```python
from build123d import *

# Parameters (mm, degrees)
F1_DEPTH      = 400
F2_W          = 150
F2_H          = 5
F2_W_2        = 75
F3_DEPTH      = 645
F4_W          = 2.5
F4_H          = 50
F5_DEPTH      = 21
F6_R          = 2
F8_DEPTH      = 143
F8_DEPTH_BACK = 143
F9_R          = 2


with BuildPart() as f1:
    # F0 (on Front) → F1 (new body)
    with BuildSketch(Plane.XZ):
        with BuildLine():
            ThreePointArc((150, 73), (148.6819805153, 76.1819805153), (145.5, 77.5))
            Line((145.5, 77.5), (0, 77.5))
            Line((0, 77.5), (-145.5, 77.5))
            ThreePointArc((-145.5, 77.5), (-148.6819805153, 76.1819805153), (-150, 73))
            Line((-150, 73), (-150, 25.5))
            ThreePointArc((-150, 25.5), (-149.7286167935, 23.960909355), (-148.947199994, 22.6074557564))
            Line((-148.947199994, 22.6074557564), (-148.5848888922, 22.1756701992))
            ThreePointArc((-148.5848888922, 22.1756701992), (-148.150768448, 21.4237515333), (-148, 20.5687011749))
            Line((-148, 20.5687011749), (-148, -77.5))
            Line((-148, -77.5), (-146, -77.5))
            Line((-146, -77.5), (-146, 20.5687011749))
            ThreePointArc((-146, 20.5687011749), (-146.2713832065, 22.1077918199), (-147.052800006, 23.4612454185))
            Line((-147.052800006, 23.4612454185), (-147.4151111078, 23.8930309758))
            ThreePointArc((-147.4151111078, 23.8930309758), (-147.849231552, 24.6449496417), (-148, 25.5))
            Line((-148, 25.5), (-148, 73))
            ThreePointArc((-148, 73), (-147.267766953, 74.767766953), (-145.5, 75.5))
            Line((-145.5, 75.5), (0, 75.5))
            Line((0, 75.5), (145.5, 75.5))
            ThreePointArc((145.5, 75.5), (147.267766953, 74.767766953), (148, 73))
            Line((148, 73), (148, 25.5))
            ThreePointArc((148, 25.5), (147.849231552, 24.6449496417), (147.4151111078, 23.8930309758))
            Line((147.4151111078, 23.8930309758), (147.052800006, 23.4612454185))
            ThreePointArc((147.052800006, 23.4612454185), (146.2713832065, 22.1077918199), (146, 20.5687011749))
            Line((146, 20.5687011749), (146, -77.5))
            Line((146, -77.5), (148, -77.5))
            Line((148, -77.5), (148, 20.5687011749))
            ThreePointArc((148, 20.5687011749), (148.150768448, 21.4237515333), (148.5848888922, 22.1756701992))
            Line((148.5848888922, 22.1756701992), (148.947199994, 22.6074557564))
            ThreePointArc((148.947199994, 22.6074557564), (149.7286167935, 23.960909355), (150, 25.5))
            Line((150, 25.5), (150, 73))
        make_face()
    extrude(amount=F1_DEPTH)

    # F2 (on face) → F3 (cut)
    with BuildSketch(Plane.YZ.offset(148)):
        with Locations((-200, -75)):
            Rectangle(F2_W, F2_H)
        with Locations((-37.5, -75)):
            Rectangle(F2_W_2, F2_H)
        with Locations((-362.5, -75)):
            Rectangle(F2_W_2, F2_H)
    extrude(amount=-F3_DEPTH, mode=Mode.SUBTRACT)

    # F4 (on face) → F5 (cut)
    with BuildSketch(Plane.XY.offset(77.5)):
        with Locations((146.75, -100)):
            Rectangle(F4_W, F4_H)
        with Locations((146.75, -300)):
            Rectangle(F4_W, F4_H)
        with Locations((-146.75, -100)):
            Rectangle(F4_W, F4_H)
        with Locations((-146.75, -300)):
            Rectangle(F4_W, F4_H)
    extrude(amount=-F5_DEPTH, mode=Mode.SUBTRACT)

    # F6
    f6_edges = [f1.edges().sort_by_distance(p)[0] for p in [
        (147, -125, -72.5),
        (147, -325, -72.5),
        (-147, -325, -72.5),
        (-147, -125, -72.5),
        (147, -75, -72.5),
        (147, -275, -72.5),
        (-147, -275, -72.5),
        (-147, -75, -72.5),
        (147, -325, -77.5),
        (147, -125, -77.5),
        (-147, -325, -77.5),
        (-147, -125, -77.5),
        (147, -275, -77.5),
        (147, -75, -77.5),
        (-147, -275, -77.5),
        (-147, -75, -77.5),
    ]]
    fillet(f6_edges, radius=F6_R)

    # F7 (on Right) → F8 (join, two sides)
    with BuildSketch(Plane.YZ) as f8_sk:
        with BuildLine():
            Line((1, 77.5), (0, 77.5))
            Line((0, 77.5), (0, 75.5))
            Line((0, 75.5), (1, 75.5))
            ThreePointArc((1, 75.5), (2.767766953, 74.767766953), (3.5, 73))
            Line((3.5, 73), (3.5, 72))
            Line((3.5, 72), (5.5, 72))
            Line((5.5, 72), (5.5, 73))
            ThreePointArc((5.5, 73), (4.1819805153, 76.1819805153), (1, 77.5))
        make_face()
    extrude(amount=F8_DEPTH)
    extrude(f8_sk.sketch, amount=-F8_DEPTH_BACK)

    # F9 (call 1 of 4: OpenCascade refuses the feature's edges together)
    f9_edges = [f1.edges().sort_by_distance(p)[0] for p in [
        (143, 0, 76.5),
    ]]
    fillet(f9_edges, radius=F9_R)

    # F9#2 (call 2 of 4)
    f9_2_edges = [f1.edges().sort_by_distance(p)[0] for p in [
        (-143, 0, 76.5),
    ]]
    fillet(f9_2_edges, radius=F9_R)

    # F9#3 (call 3 of 4)
    f9_3_edges = [f1.edges().sort_by_distance(p)[0] for p in [
        (-143, 4.5, 72),
    ]]
    fillet(f9_3_edges, radius=F9_R)

    # F9#4 (call 4 of 4)
    f9_4_edges = [f1.edges().sort_by_distance(p)[0] for p in [
        (143, 4.5, 72),
    ]]
    fillet(f9_4_edges, radius=F9_R)


solid = f1.part
```
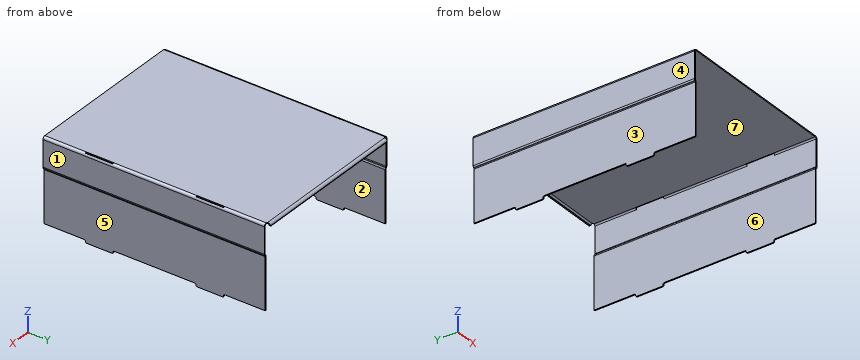
For this review, take the finished solid that the model builds, in its own axes (mm). Face numbers are marked on the shaded views. A direction names the side the tool comes from. Round coordinates to 2 decimals unless told otherwise and drop trailing zeros. Write each loop counter-clockwise with the first axis right and the second up, starting at its lowest first coordinate (ties: lowest second). Pieces come first, ordered by that corner, then holes. Notation, with made-up numbers: (45, 56) - (54, 56) arc R25 ccw to (54, 83) - close; hole circle Ø4 at (82, 51.5). An arc over 180 degrees is marked (long way). Answer as CSV lines item,"result". Start each with the question number.
(1) Add section D-D, the plane y = -183.5. State the section outline as (x, z) points, plus the area to 3 significant figures.
(2) Machinability: for the marked faces 4, 5, 6 and 7, which of the approach directions +Z, -Z, +X, -X, +Y, -Y give a long, thin tool a straight path to every point of the face, cutting with its end or side? Answer none if there is none.
(3) For pin 1 (2 mm diameter, centred on y = -72.5, z = -8, fed in from -X); pin 2 (1.6 mm diameter, centred on x = 147, y = -353.5, fed in from -Z); pin 3 (12 mm diameter, centred on y = -124, z = -27.5, fed in from +X), all flat-tipped, find the tip position at first contact; note any pin that passes through.
(4) Add section C-C, the plane x = 46. State the section outline as (y, z) points, plus the area to 3 significant figures.
(5) For line 1 (X direction, y = -353.5, z = -40.5); line 2 (X direction, y = -75, z = 30.5); line 3 (Z direction, x = -123, y = -76), list the stretches that pass through material, from the lowest coordinate up.
(6) Add section B-B, the plane y = -291. State the section outline as (x, z) points.
(7) Mouldability with a two-part tool opening along X and no side actions: class the marked faces 1, 2 and 3 as +X half, -X half, draft (parallel to the pull), parting line (faces both ways), or undercut.
(8) Add section A-A, the plane z = 59.5. State the section outline as (x, y) points.
From the geometry:
1,outline,"(-150, 25.5) arc R4.5 ccw to (-148.95, 22.61) - (-148.58, 22.18) arc R2.5 cw to (-148, 20.57) - (-148, -72.5) - (-146, -72.5) - (-146, 20.57) arc R4.5 ccw to (-147.05, 23.46) - (-147.42, 23.89) arc R2.5 cw to (-148, 25.5) - (-148, 73) arc R2.5 cw to (-145.5, 75.5) - (145.5, 75.5) arc R2.5 cw to (148, 73) - (148, 25.5) arc R2.5 cw to (147.42, 23.89) - (147.05, 23.46) arc R4.5 ccw to (146, 20.57) - (146, -72.5) - (148, -72.5) - (148, 20.57) arc R2.5 cw to (148.58, 22.18) - (148.95, 22.61) arc R4.5 ccw to (150, 25.5) - (150, 73) arc R4.5 ccw to (145.5, 77.5) - (-145.5, 77.5) arc R4.5 ccw to (-150, 73) - close"
1,area,"1,190 mm²"
2,face 4,"+Z, -Z, -X, +Y, -Y"
2,face 5,"-Z, +X, +Y, -Y"
2,face 6,"-Z, +Y, -Y"
2,face 7,"-Z, -Y"
3,pin 1,"stops at x = -148"
3,pin 2,"stops at z = -72.5"
3,pin 3,"stops at x = 148"
4,outline,"(-400, 75.5) - (1, 75.5) arc R2.5 cw to (3.5, 73) - (3.5, 72) - (5.5, 72) - (5.5, 73) arc R4.5 ccw to (1, 77.5) - (-400, 77.5) - close"
4,area,"815 mm²"
5,line 1,"x = -148 to -146, 146 to 148"
5,line 2,"x = -150 to -148, 148 to 150"
5,line 3,"z = 75.5 to 77.5"
6,outline,"(-150, 25.5) arc R4.5 ccw to (-148.95, 22.61) - (-148.58, 22.18) arc R2.5 cw to (-148, 20.57) - (-148, -77.5) - (-146, -77.5) - (-146, 20.57) arc R4.5 ccw to (-147.05, 23.46) - (-147.42, 23.89) arc R2.5 cw to (-148, 25.5) - (-148, 76.74) arc R4.5 ccw to (-150, 73) - close; (-145.5, 75.5) - (145.5, 75.5) - (145.5, 77.5) - (-145.5, 77.5) - close; (146, -77.5) - (148, -77.5) - (148, 20.57) arc R2.5 cw to (148.58, 22.18) - (148.95, 22.61) arc R4.5 ccw to (150, 25.5) - (150, 73) arc R4.5 ccw to (148, 76.74) - (148, 25.5) arc R2.5 cw to (147.42, 23.89) - (147.05, 23.46) arc R4.5 ccw to (146, 20.57) - close"
7,face 1,"+X half"
7,face 2,"undercut"
7,face 3,"-X half"
8,outline,"(-150, -400) - (-148, -400) - (-148, 0) - (-150, 0) - close; (148, -400) - (150, -400) - (150, 0) - (148, 0) - close"
